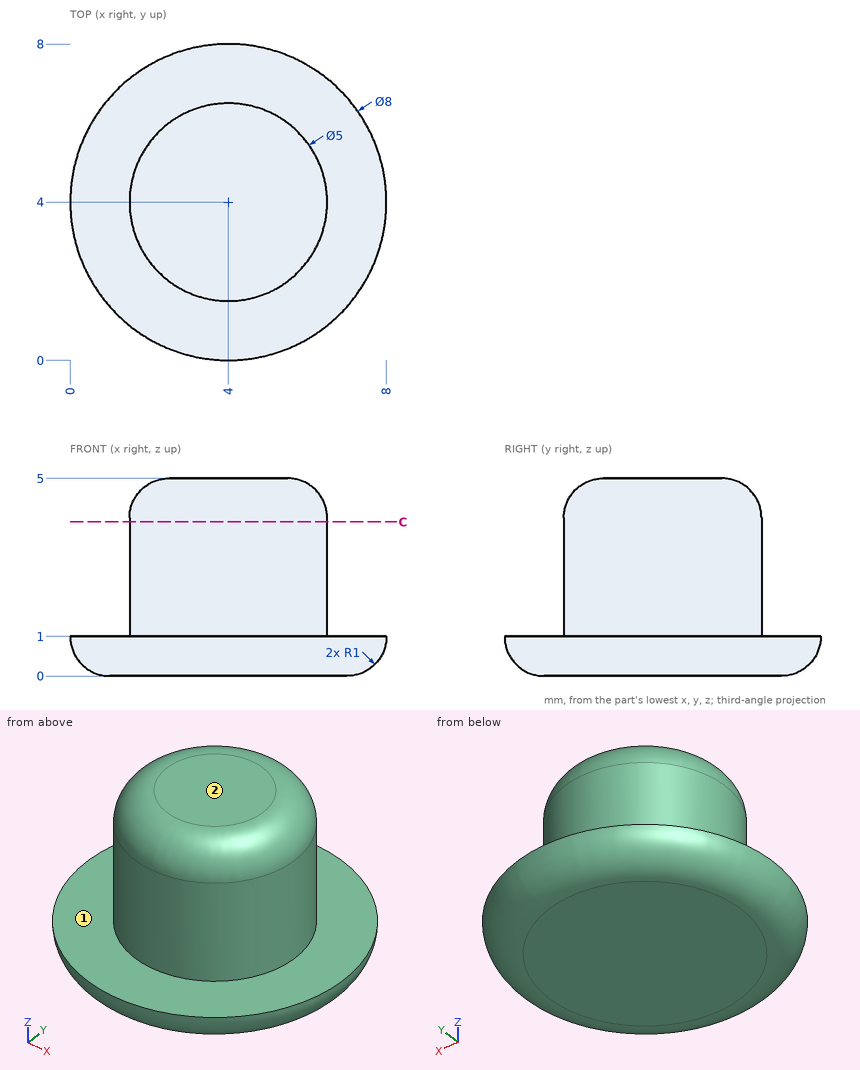
Drawing for the job (mm, zero at the part's lowest x, y, z). A direction names the side the tool comes from. Round coordinates to 2 decimals unless told otherwise and drop trailing zeros. Order: outer loops, then holes, each group sorted by start corner. A loop starts at its lowest first (then second) coordinate and runs counter-clockwise, first axis right, second up. Notation, with made-up numbers: M -29,7 L 17,7 A28 cw 17,39 Z; hole C 10.5,-5.75 d2. An arc over 180 degrees is marked long. Use one line per item in the form item = value.
Q1. Saw through at C-C on z = 3.9. Give the cut face in (x, y).
Recorded:
outline = C 4,4 d5
Q2. Flat gauge pin, fed straight in: P1, Ø2, axis at x = 5.5, z = 4.5, coming from the +Y side. Where does the tip first touch, or does it go through?
Recorded:
P1 = 6.43
Q3. Which spindle directions (+Z, -Z, +X, -X, +Y, -Y) get a long thin tool onto all of the face, cutting with end or side? Do the marked faces 1 and 2. Say none if no direction does.
Recorded:
face_1 = +Z
face_2 = +Z, +X, -X, +Y, -Y
Q4. Probe L1, parallel to Z at x = 2, y = 6; L2, parallel to X at y = 6, z = 3.95; L3, parallel to Z at x = 5.25, y = 5.25. List the from-to ranges inside material, lowest first.
Recorded:
L1 = 0 to 1
L2 = 2.5 to 5.5
L3 = 0 to 4.96
